Input: part model. Units: mm. Frame: model coordinates. Give positions to 0.01 mm unless a question says otherwise; leave off trailing zeros. Write each loop counter-clockwise with the first axis right and the second up, starting at its lowest first coordinate (ties: lowest second). Pieces come first, ordered by that corner, then holes. Notation, with made-up numbers: (52, 45) - (93, 45) arc R9 ccw to (93, 62) - close; hole circle Ø11 at (-6, 71). An arc over 180 degrees is marked (long way). Use a Markdown table: item, result. Add a question column.
1. Section query A-A, the plane z = 0. Return loops of the section in (x, y), plus the area to 3 significant figures.
2. Pin query (flat end, axial travel): pin 1 (6 mm diameter, centred on x = 27.5, z = 0, fed in from -Y); pin 2 (1 mm diameter, centred on y = 3.5, z = -26, fed in from +X); pin 3 (2 mm diameter, centred on x = -37.5, y = 2, fed in from +Z); pin 4 (1.2 mm diameter, centred on x = 37, y = 2.5, fed in from -Z). Return the tip coordinate at first contact, or that it passes through.
3. Section query D-D, the plane z = 31. Return loops of the section in (x, y), plus the area to 3 significant figures.
4. Section query C-C, the plane z = 16. Return loops of the section in (x, y).
5. Section query B-B, the plane y = 0.6. Return loops of the section in (x, z).
6. Material intervals for probe 1 along X at (y, z) = (1.7, 0); probe 2 along X at (y, z) = (1.5, 14.5); probe 3 along Z at (x, y) = (36.5, 0.85), sorted ascending.
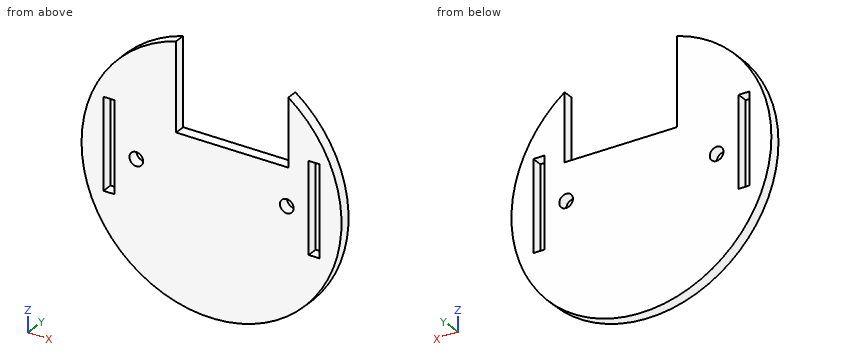
```python
from build123d import *

# Parameters (mm, degrees)
SKETCH1_R           = 2.5
BOSS_EXTRUDE2_DEPTH = 4


with BuildPart() as part:
    # Sketch1 → Boss-Extrude2 (new body)
    with BuildSketch(Plane(origin=(0, 0, 0), x_dir=(1, 0, 0), z_dir=(0, 1, 0))):
        with BuildLine():
            Line((-12.928995443, -45.70657586), (-12.928995443, -13.70657586))
            Line((-12.928995443, -13.70657586), (28.071004557, -13.70657586))
            Line((28.071004557, -13.70657586), (28.071004557, -38.317994509))
            ThreePointArc((28.071004557, -38.317994509), (-8.424244393, 46.747001042), (-12.928995443, -45.70657586))
        make_face()
        with Locations(Location((-27.5, 0, 0), (0, 0, 270))):
            Circle(SKETCH1_R, mode=Mode.SUBTRACT)
        with Locations(Location((27.5, 0, 0), (0, 0, 90))):
            Circle(SKETCH1_R, mode=Mode.SUBTRACT)
        Polygon((35.5, -18.298658927), (39.5, -18.298658927), (39.5, 14.701341073), (35.5, 14.701341073), (35.5, 9.151429429), align=None, mode=Mode.SUBTRACT)
        Polygon((-35.5, -18.298658927), (-39.5, -18.298658927), (-39.5, 14.701341073), (-35.5, 14.701341073), (-35.5, 9.151429429), align=None, mode=Mode.SUBTRACT)
    extrude(amount=BOSS_EXTRUDE2_DEPTH)


solid = part.part
```
Result sheet:
| question | item | result |
|---|---|---|
| 1 | outline | (-47.5, 0) - (-39.5, 0) - (-39.5, 4) - (-47.5, 4) - close; (-35.5, 0) - (-30, 0) - (-30, 4) - (-35.5, 4) - close; (-25, 0) - (25, 0) - (25, 4) - (-25, 4) - close; (30, 0) - (35.5, 0) - (35.5, 4) - (30, 4) - close; (39.5, 0) - (47.5, 0) - (47.5, 4) - (39.5, 4) - close |
| 1 | area | 308 mm² |
| 2 | pin 1 | stops at y = 0 |
| 2 | pin 2 | stops at x = 40.07 |
| 2 | pin 3 | stops at z = 30.4 |
| 2 | pin 4 | stops at z = -30.52 |
| 3 | outline | (-35.99, 0) - (-12.93, 0) - (-12.93, 4) - (-35.99, 4) - close; (28.07, 0) - (35.99, 0) - (35.99, 4) - (28.07, 4) - close |
| 3 | area | 124 mm² |
| 4 | outline | (-44.72, 0) - (-39.5, 0) - (-39.5, 4) - (-44.72, 4) - close; (-35.5, 0) - (-12.93, 0) - (-12.93, 4) - (-35.5, 4) - close; (28.07, 0) - (35.5, 0) - (35.5, 4) - (28.07, 4) - close; (39.5, 0) - (44.72, 0) - (44.72, 4) - (39.5, 4) - close |
| 5 | outline | (-12.93, 13.71) - (-12.93, 45.71) arc R47.5 ccw (long way) to (28.07, 38.32) - (28.07, 13.71) - close; hole (-39.5, -14.7) - (-35.5, -14.7) - (-35.5, 18.3) - (-39.5, 18.3) - close; hole circle Ø5 at (-27.5, 0); hole circle Ø5 at (27.5, 0); hole (35.5, -14.7) - (39.5, -14.7) - (39.5, 18.3) - (35.5, 18.3) - close |
| 6 | probe 1 | x = -47.5 to -39.5, -35.5 to -30, -25 to 25, 30 to 35.5, 39.5 to 47.5 |
| 6 | probe 2 | x = -45.23 to -39.5, -35.5 to -12.93, 28.07 to 35.5, 39.5 to 45.23 |
| 6 | probe 3 | z = -30.4 to -14.7, 18.3 to 30.4 |
